Can you work these out from the drawing? Everything is in mm from the part's minimum corner. Round coordinates to 2 decimals unless told otherwise and drop trailing zeros. Write each loop counter-clockwise with the first axis right and the second up, starting at its lowest first coordinate (ties: lowest second). Pieces come first, ordered by that corner, then holes. Notation, with made-up numbers: (4, -8) -> (22, -8) arc R22 cw to (22, 18) -> close; hole circle Ø9 at (-31, 8). An arc over 180 degrees is marked (long way). One line per question, with ' | ' between items. Start each with the question number.
1. Imagine slicing it at C-C, the plane z = 58. List the corners of the cut face in (x, y) for me, and give its area (3 significant figures).
2. For pin 1 Ø4 at (x, y) = (12.5, 14) entering from +Z; pin 2 Ø8 at (y, z) = (4, 26) entering from +X; pin 3 Ø5 at (x, z) = (15, 16.5) entering from +Y; pin 4 Ø10 at (x, z) = (3, 7) entering from -Y, each with a flat end and sliding along its axis, tell me the tip position at first contact or that it passes through.
3. Thinking about a two-plate mould opening in X: for the marked faces 1 and 2, which applies, released by +X, released by -X, zero draft, split by the parting line, or undercut?
4. If I drill on line 1 along Y through (x, z) = (8.5, 25); line 2 along Y through (x, z) = (15.25, 52); line 3 along X through (y, z) = (14.75, 18.5), over which ranges is the centre line in solid material (lowest first)? Write a range as [from, to].
5. Imagine slicing it at A-A, the plane x = 8.5. List the corners of the cut face in (y, z) for me.
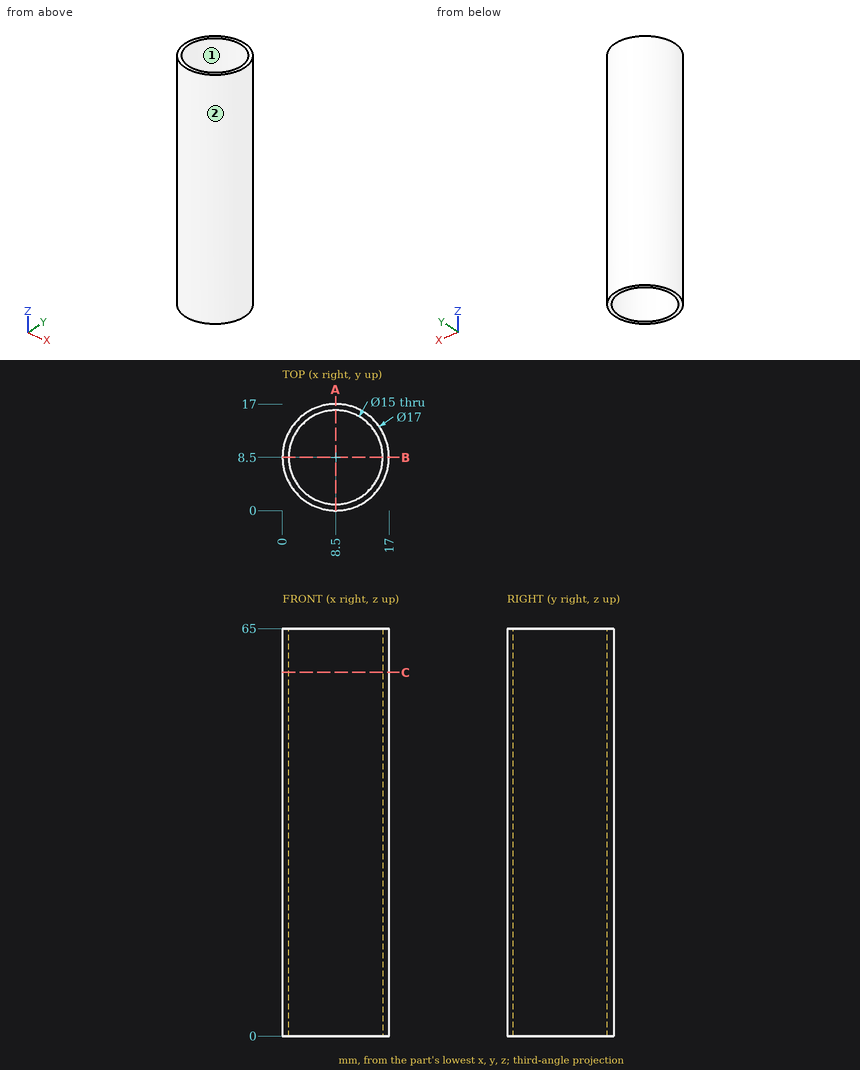
Geometry results:
1) outline: circle Ø17 at (8.5, 8.5); hole circle Ø15 at (8.5, 8.5) | area: 50.3 mm2
2) pin 1: stops at z = 65 | pin 2: stops at x = 16.99 | pin 3: stops at y = 16 | pin 4: stops at y = 0.01
3) face 1: undercut | face 2: split by the parting line
4) line 1: y = [0, 1], [16, 17] | line 2: y = [3.33, 5.23], [11.77, 13.67] | line 3: x = [2.74, 4.35], [12.65, 14.26]
5) outline: (0, 0) -> (1, 0) -> (1, 65) -> (0, 65) -> close; (16, 0) -> (17, 0) -> (17, 65) -> (16, 65) -> close
